from build123d import *

# Parameters (mm, degrees)
ESQUISSE1_W             = 12
ESQUISSE1_H             = 12
BOSS_EXTRU_1_DEPTH      = 50
ENL_V_MAT_EXTRU_1_DEPTH = 50
ESQUISSE3_R             = 3.25
ENL_V_MAT_EXTRU_2_DEPTH = 47
ESQUISSE4_R             = 1.5
ENL_V_MAT_EXTRU_3_DEPTH = 3


with BuildPart() as part:
    # Esquisse1 → Boss.-Extru.1 (new body)
    with BuildSketch(Plane(origin=(0, 0, 0), x_dir=(1, 0, 0), z_dir=(0, 1, 0))):
        Rectangle(ESQUISSE1_W, ESQUISSE1_H)
    extrude(amount=BOSS_EXTRU_1_DEPTH)

    # Esquisse2 → Enlèv. mat.-Extru.1 (cut)
    with BuildSketch(Plane(origin=(0, 50, 0), x_dir=(1, 0, 0), z_dir=(0, 1, 0))):
        Polygon((-5, -0.8), (-5, -1.8), (-4, -1.8), (-4, 1.8), (-5, 1.8), (-5, 0.8), (-6, 0.8), (-6, -0.8), align=None)
        Polygon((1.8, 5), (1.8, 4), (-1.8, 4), (-1.8, 5), (-0.8, 5), (-0.8, 6), (0.8, 6), (0.8, 5), align=None)
        Polygon((5, -1.8), (4, -1.8), (4, 1.8), (5, 1.8), (5, 0.8), (6, 0.8), (6, -0.8), (5, -0.8), align=None)
        Polygon((-1.8, -5), (-1.8, -4), (1.8, -4), (1.8, -5), (0.8, -5), (0.8, -6), (-0.8, -6), (-0.8, -5), align=None)
    extrude(amount=-ENL_V_MAT_EXTRU_1_DEPTH, mode=Mode.SUBTRACT)

    # Esquisse3 → Enlèv. mat.-Extru.2 (cut)
    with BuildSketch(Plane(origin=(0, 50, 0), x_dir=(1, 0, 0), z_dir=(0, 1, 0))):
        with Locations(Location((0, 0, 0), (0, 0, 270))):
            Circle(ESQUISSE3_R)
    extrude(amount=-ENL_V_MAT_EXTRU_2_DEPTH, mode=Mode.SUBTRACT)

    # Esquisse4 → Enlèv. mat.-Extru.3 (cut)
    with BuildSketch(Plane(origin=(0, 3, 0), x_dir=(1, 0, 0), z_dir=(0, 1, 0))):
        with Locations(Location((0, 0, 0), (0, 0, 270))):
            Circle(ESQUISSE4_R)
    extrude(amount=-ENL_V_MAT_EXTRU_3_DEPTH, mode=Mode.SUBTRACT)


solid = part.part
CAD build for the part. Positions are in the model's coordinates, mm. A direction names the side the tool comes from. Coordinates: 2 decimals unless noted, no trailing zeros. Loops run counter-clockwise (first coordinate to the right, second up) from the corner with the lowest first, then second, coordinate; pieces in that order, holes last. Notation, with made-up numbers: (83.5, -12.5) - (103.5, -12.5) arc R14 ccw to (103.5, 5.5) - close; hole circle Ø7 at (71, -7). An arc over 180 degrees is marked (long way). Write item = value, one per line. Start each with the question number.
Q1. Cut at B-B, the plane z = 0. List the corners of the cut face in (x, y), then the cut area to 3 significant figures.
Q2. Which spindle directions (+Z, -Z, +X, -X, +Y, -Y) get a long thin tool onto all of the face, cutting with end or side? Do faces 1 (the flat face through (0, 25, 4)), 2 (the flat face through (-0.8, 25.4, -5.5)), 3 (the flat face through (5.5, 25.4, -0.8)). Say none if no direction does.
Q3. Flat gauge pin, fed straight in: pin 1 Ø4 at (x, z) = (0, 0) entering from +Y. Where does the tip first touch, or does it go through?
Q4. Drill centre lines: L1, parallel to Z at x = -1.5, y = 25; L2, parallel to X at y = 39.5, z = 0; L3, parallel to X at y = 26, z = 1.25. Where is each one in solid material? Low to high.
Q5. Cut at A-A, the plane x = 0. List the corners of the cut face in (y, z), then the cut area to 3 significant figures.
Q6. Pull direction X, two halves, no side cores. Call faces 4 (the flat face through (5, 25, -1)), 5 (the flat face through (-5.5, 25.4, -0.8)), 6 (the flat face through (6, 25, 3)): pulls with the +X half, pulls with the -X half, needs draft (parallel to the pull), parting line crosses it, or undercut.
Computed:
q1.outline = (-4, 0) - (-1.5, 0) - (-1.5, 3) - (-3.25, 3) - (-3.25, 50) - (-4, 50) - close; (1.5, 0) - (4, 0) - (4, 50) - (3.25, 50) - (3.25, 3) - (1.5, 3) - close
q1.area = 85.5 mm²
q2.face_1 = +Y, -Y
q2.face_2 = -Z, +Y, -Y
q2.face_3 = +X, +Y, -Y
q3.pin_1 = 3
q4.L1 = -6 to -5, -4 to -2.88, 2.88 to 4, 5 to 6
q4.L2 = -4 to -3.25, 3.25 to 4
q4.L3 = -6 to -5, -4 to -3, 3 to 4, 5 to 6
q5.outline = (0, -4) - (50, -4) - (50, -3.25) - (3, -3.25) - (3, -1.5) - (0, -1.5) - close; (0, 1.5) - (3, 1.5) - (3, 3.25) - (50, 3.25) - (50, 4) - (0, 4) - close
q5.area = 85.5 mm²
q6.face_4 = undercut
q6.face_5 = needs draft
q6.face_6 = pulls with the +X half
